Study the drawing (mm; zero at the part's minimum x, y, z) and answer. A direction names the side the tool comes from. Coordinates: 2 decimals unless noted, no trailing zeros. Loops run counter-clockwise (first coordinate to the right, second up) from the corner with the lowest first, then second, coordinate; pieces in that order, holes last. Notation, with made-up numbers: (-40, 30.25) -> (-32, 30.25) arc R26 cw to (-32, 62.25) -> close; hole circle Ø2 at (-6, 68). An arc over 180 degrees is marked (long way). Answer in a Markdown table with one row per item.
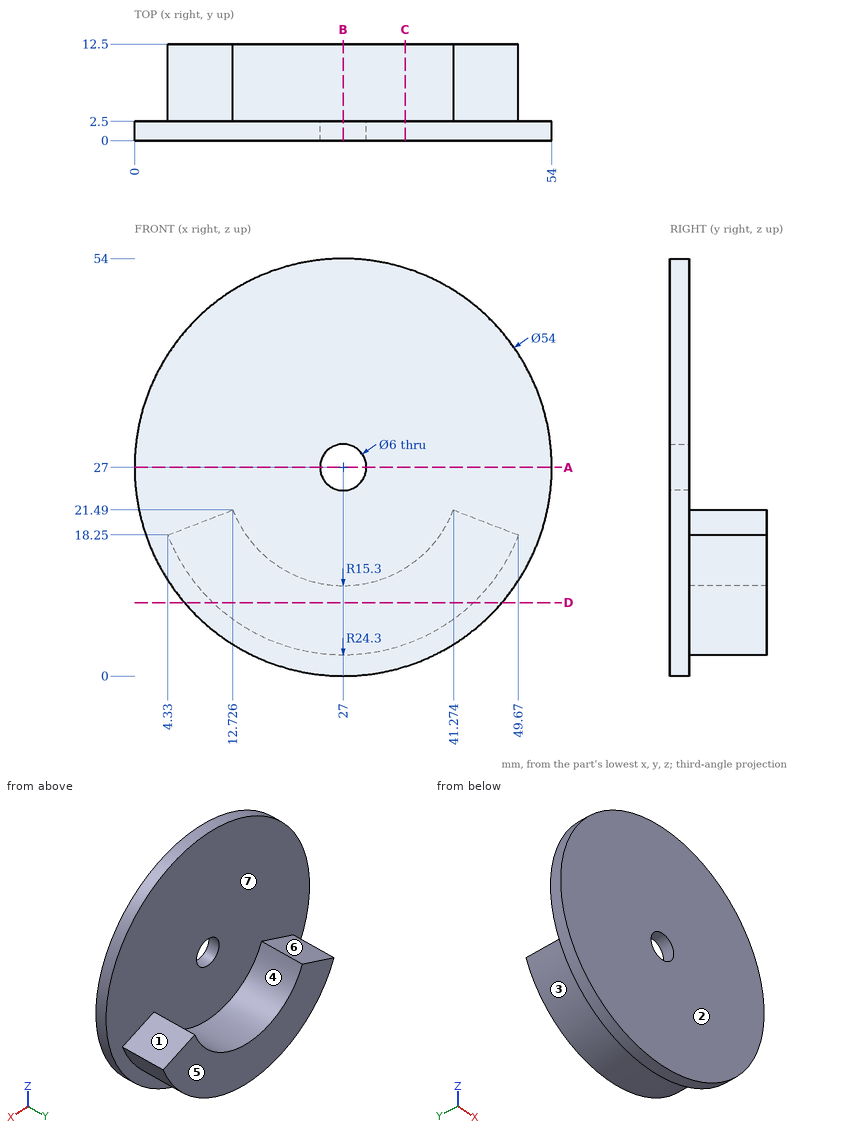
1. Given pin 1 Ø1.5 at (x, z) = (35, 46.5) entering from -Y; pin 2 Ø5 at (x, y) = (16.5, 9) entering from +Z; pin 3 Ø7 at (x, z) = (27, 27) entering from +Y; pin 4 Ø1 at (y, z) = (3.5, 42.5) entering from +X, each flat-ended and moving along its own axis, determine where each tip first touches the part or whether it passes through.
A:
| item | result |
|---|---|
| pin 1 | stops at y = 0 |
| pin 2 | stops at z = 18.93 |
| pin 3 | stops at y = 2.5 |
| pin 4 | passes through |
2. A cutting plane is placed at D-D on z = 9.5. Give the vertices of the cut face in (x, y).
A:
| item | result |
|---|---|
| outline | (6.44, 0) -> (47.56, 0) -> (47.56, 2.5) -> (43.86, 2.5) -> (43.86, 12.5) -> (10.14, 12.5) -> (10.14, 2.5) -> (6.44, 2.5) -> close |
3. A cutting plane is placed at C-C on x = 35. Give the vertices of the cut face in (y, z) (1 decimal).
A:
| item | result |
|---|---|
| outline | (0, 1.2) -> (2.5, 1.2) -> (2.5, 4.1) -> (12.5, 4.1) -> (12.5, 14) -> (2.5, 14) -> (2.5, 52.8) -> (0, 52.8) -> close |
4. A tool of negligible diameter and unlimited length cuts with its end or side. For the marked faces 1, 2 and 3, from which of +Z, -Z, +X, -X, +Y, -Y can it reach the whole face along a straight path? Write none if from no direction.
A:
| item | result |
|---|---|
| face 1 | +Z, +X, +Y |
| face 2 | +Z, -Z, +X, -X, -Y |
| face 3 | -Z, +Y |
5. The mould has two halves that part along X. Classify the marked faces 4, 5, 6 and 7: pulls with the +X half, pulls with the -X half, needs draft (parallel to the pull), parting line crosses it, or undercut.
A:
| item | result |
|---|---|
| face 4 | undercut |
| face 5 | needs draft |
| face 6 | pulls with the -X half |
| face 7 | undercut |
6. A cutting plane is placed at B-B on x = 27. Give the vertices of the cut face in (y, z).
A:
| item | result |
|---|---|
| outline | (0, 0) -> (2.5, 0) -> (2.5, 2.7) -> (12.5, 2.7) -> (12.5, 11.7) -> (2.5, 11.7) -> (2.5, 24) -> (0, 24) -> close; (0, 30) -> (2.5, 30) -> (2.5, 54) -> (0, 54) -> close |
7. A cutting plane is placed at A-A on z = 27. Give the vertices of the cut face in (x, y), and give its area (3 significant figures).
A:
| item | result |
|---|---|
| outline | (0, 0) -> (24, 0) -> (24, 2.5) -> (0, 2.5) -> close; (30, 0) -> (54, 0) -> (54, 2.5) -> (30, 2.5) -> close |
| area | 120 mm2 |
8. Find the intervals of material crossed by probe 1 along X at (y, z) = (1.7, 27); probe 2 along Y at (x, z) = (49, 16); probe 3 along Z at (x, y) = (27.5, 8.5) (1 decimal), in increasing order.
A:
| item | result |
|---|---|
| probe 1 | x = 0 to 24, 30 to 54 |
| probe 2 | y = 0 to 2.5 |
| probe 3 | z = 2.7 to 11.7 |
